Autodesk Inventor part; units mm, degrees
ref_plane "YZ Plane" through (0, 0, 0) normal (1, 0, 0) x (0, 1, 0)
ref_plane "XZ Plane" through (0, 0, 0) normal (0, 1, 0) x (-1, 0, 0)
ref_plane "XY Plane" through (0, 0, 0) normal (0, 0, 1) x (1, 0, 0)
sketch "Sketch1" plane through (0, 0, 0) normal (0, 1, 0) x (-1, 0, 0)
  line L0 (0, 0) -> (50, 0)
  line L1 (50, 0) -> (50, -60)
  line L2 (50, -60) -> (0, -60)
  line L3 (0, -60) -> (0, 0)
  dimension "d0" = 50
  dimension "d1" = 60
extrude "Extrusion1" add sketch "Sketch1" along normal blind 5
sketch "Sketch2" plane through (0, 5, 0) normal (0, 1, 0) x (1, 0, 0)
  line L0 (-50, 0) -> (0, 0)
  line L1 (-50, 60) -> (-50, 0)
  line L2 (0, 0) -> (-50, 0)
  line L3 (-50, 0) -> (-50, 40)
  line L4 (-50, 40) -> (0, 40)
  line L5 (0, 40) -> (0, 0)
  dimension "d4" = 40
extrude "Extrusion2" add sketch "Sketch2" along normal blind 11
sketch "Sketch3" plane through (0, 16, 0) normal (0, 1, 0) x (1, 0, 0)
  line L0 (0, 0) -> (-50, 0)
  line L1 (-50, 0) -> (-50, 60)
  line L2 (-50, 60) -> (0, 60)
  line L3 (0, 60) -> (0, 0)
extrude "Extrusion3" add sketch "Sketch3" along normal blind 5
sketch "Sketch4" plane through (0, 21, 0) normal (0, 1, 0) x (1, 0, 0)
  line L0 (0, 0) -> (0, 60)
  line L1 (-50, 40) -> (0, 40)
  line L2 (0, 60) -> (-50, 60)
  line L3 (-50, 60) -> (-50, 40)
  line L4 (-50, 40) -> (0, 40)
  line L5 (0, 40) -> (0, 60)
  line L6 (-50, 50) -> (0, 50)
  line L7 (-25, 50) -> (-50, 50)
  line L8 (-25, 50) -> (0, 50)
  circle A0 centre (-12.5, 50) radius 2.5
  circle A1 centre (-37.5, 50) radius 2.5
  dimension "d9" = 5
  dimension "d10" = 5
extrude "Extrusion4" cut sketch "Sketch4" against normal blind 5 contours A0 L6 | L6 A0 | A1 L6 | L6 A1
sketch "Sketch5" plane through (0, 21, 0) normal (0, 1, 0) x (1, 0, 0)
  line L0 (-50, 60) -> (-50, 0)
  line L1 (0, 0) -> (-50, 0)
  line L2 (-50, 0) -> (-50, 35)
  line L3 (-50, 35) -> (0, 35)
  line L4 (0, 35) -> (0, 0)
  line L5 (-37.5, 35) -> (-37.5, 0)
  line L6 (-12.5, 35) -> (-12.5, 0)
  dimension "d13" = 35
extrude "Extrusion5" add sketch "Sketch5" along normal blind 30 contours L3 L6 L1 L5
sketch "Sketch6" plane through (0, 51, 0) normal (0, 1, 0) x (1, 0, 0)
  line L0 (0, 0) -> (0, 60)
  line L1 (0, 0) -> (-49.8487, 0)
  line L2 (-49.8487, 0) -> (-49.8487, 35.2322)
  line L3 (-49.8487, 35.2322) -> (0, 35.2322)
  line L4 (0, 35.2322) -> (0, 0)
  line L5 (-49.8487, 17.6161) -> (0, 17.6161) construction
  line L6 (-24.9244, 0) -> (-24.9244, 35.2322) construction
  circle A0 centre (-24.9244, 17.6161) radius 5
  dimension "d16" = 10
extrude "Extrusion6" cut sketch "Sketch6" against normal blind 30 contours A0
sketch "Sketch7" plane through (0, 51, 0) normal (0, 1, 0) x (1, 0, 0)
  line L0 (-50, 35) -> (-50, 0)
  line L1 (0, 0) -> (-50, 0)
  line L2 (-50, 0) -> (-50, 35)
  line L3 (-50, 35) -> (0, 35)
  line L4 (0, 35) -> (0, 0)
  circle A0 centre (-24.9244, 17.6161) radius 5
  circle A1 centre (-24.9244, 17.6161) radius 5
  line L5 (-37.5, 35) -> (-37.5, 0)
  line L6 (-12.5, 35) -> (-12.5, 0)
extrude "Extrusion7" add sketch "Sketch7" along normal blind 10 contours L3 L6 L1 L5
chamfer "Chamfer1" distance 4 angle 45 1 edges at (-29.9244, 61, -17.6161)
sketch "Sketch8" plane through (0, 0, 0) normal (0, -1, 0) x (1, 0, 0)
  point P0 (0, 0)
sketch "Sketch9" plane through (0, 0, 0) normal (0, -1, 0) x (1, 0, 0)
  line L0 (0, -60) -> (-50, -60)
  line L1 (0, -60) -> (-15, -60)
  line L2 (-15, -60) -> (-15, -45)
  line L3 (-15, -45) -> (0, -45)
  line L4 (0, -45) -> (0, -60)
  line L5 (-50, -60) -> (-50, 0)
  line L6 (-50, -60) -> (-35, -60)
  line L7 (-35, -60) -> (-35, -45)
  line L8 (-35, -45) -> (-50, -45)
  line L9 (-50, -45) -> (-50, -60)
  line L10 (0, 0) -> (-15, 0)
  line L11 (-15, 0) -> (-15, -15)
  line L12 (-15, -15) -> (0, -15)
  line L13 (0, -15) -> (0, 0)
  line L14 (-50, 0) -> (-35, 0)
  line L15 (-35, 0) -> (-35, -15)
  line L16 (-35, -15) -> (-50, -15)
  line L17 (-50, -15) -> (-50, 0)
  point P0 (-50, -35)
  dimension "d24" = 15
  dimension "d25" = 15
  dimension "d26" = 15
  dimension "d27" = 15
  dimension "d28" = 15
  dimension "d29" = 15
extrude "Extrusion8" add sketch "Sketch9" along normal blind 12
fillet "Fillet1" radius 2 7 edges at (-25, 61, -35) (-25, 61, 0) (-25, 21, -60) (-25, 16, -60) (-25, 5, -60) (-12.5, 61, -17.5) (-37.5, 61, -17.5)
fillet "Fillet2" radius 1 10 edges at (-50, 20.4142, -59.4142) (-50, 18.5, -60) (-50, 16.5858, -59.4142) (-50, 16, -49) (-50, 21, -29) (0, 20.4142, -59.4142) (0, 18.5, -60) (0, 16.5858, -59.4142) (0, 16, -49) (0, 21, -29)
fillet "Fillet3" radius 1 16 edges at (-49.7071, 20.7071, 0) (-50, 4, 0) (-43.25, 21, 0) (-0.2929, 20.7071, 0) (0, 4, 0) (-6.75, 21, 0) (-50, 4.4142, -59.4142) (-50, 5, -49) (-50, -4.5, -60) (0, 4.4142, -59.4142) (0, 5, -49) (0, -4.5, -60) (0, 16.5, -40) (0, 10.5, -40) (-50, 16.5, -40) (-50, 10.5, -40)
fillet "Fillet4" radius 1 15 edges at (-13.0858, 60.4142, -0.5858) (-12.5, 40, 0) (-12.5, 20.5, 0) (-36.9142, 60.4142, -0.5858) (-37.5, 20.5, 0) (-37.5, 40, 0) (-13.0858, 60.4142, -34.4142) (-12.5, 40, -35) (-36.9142, 60.4142, -34.4142) (-37.5, 40, -35) (-37.5, 20.7071, -0.2929) (-37.5, 21, -18) (-25, 21, -35) (-12.5, 20.7071, -0.2929) (-12.5, 21, -18)
properties part number "PortaHerramienta1"
Read the model definition and answer for the solid it produces. Units are mm, in the model's axes. A direction names the side the tool comes from. Round coordinates to 2 decimals unless told otherwise and drop trailing zeros. Write each loop counter-clockwise with the first axis right and the second up, starting at its lowest first coordinate (ties: lowest second). Pieces come first, ordered by that corner, then holes. Notation, with made-up numbers: (25, -35.5) - (39, -35.5) arc R22 cw to (39, -15.5) - close; hole circle Ø1 at (89.25, 66). An arc over 180 degrees is marked (long way). One line per item, written item: value.
Q1. Find section A-A (z = -50). Determine the outline of the cut face in (x, y), and give its area (3 significant figures).
The answers:
outline: (-50, -12) - (-35, -12) - (-35, 0) - (-15, 0) - (-15, -12) - (0, -12) - (0, 4) arc R1 ccw to (-1, 5) - (-49, 5) arc R1 ccw to (-50, 4) - close; (-50, 17) arc R1 ccw to (-49, 16) - (-40, 16) - (-40, 21) - (-49, 21) arc R1 ccw to (-50, 20) - close; (-35, 16) - (-15, 16) - (-15, 21) - (-35, 21) - close; (-10, 16) - (-1, 16) arc R1 ccw to (0, 17) - (0, 20) arc R1 ccw to (-1, 21) - (-10, 21) - close
area: 809 mm2
Q2. Find section B-B (y = -7). Determine the outline of the cut face in (x, z), and give its area (3 significant figures).
The answers:
outline: (-50, -59) arc R1 ccw to (-49, -60) - (-35, -60) - (-35, -45) - (-50, -45) - close; (-50, -15) - (-35, -15) - (-35, 0) - (-49, 0) arc R1 ccw to (-50, -1) - close; (-15, -60) - (-1, -60) arc R1 ccw to (0, -59) - (0, -45) - (-15, -45) - close; (-15, -15) - (0, -15) - (0, -1) arc R1 ccw to (-1, 0) - (-15, 0) - close
area: 899 mm2
Q3. Which of the six approach directions +Z, -Z, +X, -X, +Y, -Y give full straight-line access (tool end or side, diameter ignored) to faces 5 (the cylindrical face through (-24.66, 4.4, -59.43)), 6 (the flat face through (-8, -6, -45)), 7 (the flat face through (-25, 40, -35)), 8 (the cylindrical face through (-35.19, 18.54, -49.04))?
The answers:
face 5: -Z, +X, -X
face 6: +X, -X, -Y
face 7: -Z, +X, -X, +Y
face 8: +Y
Q4. Each of these flat-tipped pins is pushed along its axis until it touches: P1, Ø8, axis at x = -24.92, z = -17.62, coming from the -Y side; P2, Ø5.5, axis at x = -34.5, z = -48.5, coming from the +Y side; P3, Ø9, axis at x = -16.5, y = 8.5, coming from the -Z side. Where does it stop, or does it pass through?
The answers:
P1: stops at y = 0
P2: stops at y = 21
P3: stops at z = -59.73
Q5. For a pull along Y with two mould halves and no side action, classify faces 1 (the cylindrical face through (-24.66, 16.57, -59.4)), 2 (the flat face through (-25, 16, -49)), 3 (the flat face through (-50, 4, -30)), 4 (the flat face through (-25.3, 21, -36.2)) as pulls with the +Y half, pulls with the -Y half, needs draft (parallel to the pull), parting line crosses it, or undercut.
The answers:
face 1: undercut
face 2: undercut
face 3: needs draft
face 4: pulls with the +Y half
Q6. Find section D-D (x = -43.5). Determine the outline of the cut face in (y, z), and give its area (3 significant figures).
The answers:
outline: (-12, -60) - (3, -60) arc R2 ccw to (5, -58) - (5, -40) - (16, -40) - (16, -58) arc R2 ccw to (18, -60) - (19, -60) arc R2 ccw to (21, -58) - (21, -1) arc R1 ccw to (20, 0) - (-12, 0) - (-12, -15) - (0, -15) - (0, -45) - (-12, -45) - close
area: 1,400 mm2
Q7. Straight lines are drawn through the part: line 1 (X direction, y = 19, z = -50); line 2 (Z direction, x = -5, y = -3.5); line 3 (Y direction, x = -40, z = -46.5). For each, find the intervals that lie inside material, in ascending order. Write a range as from..to.
The answers:
line 1: x = -50..-40, -35..-15, -10..0
line 2: z = -60..-45, -15..0
line 3: y = -12..5, 16..21
Q8. Find section C-C (z = -43). Determine the outline of the cut face in (x, y).
The answers:
outline: (-50, 0) - (0, 0) - (0, 4) arc R1 ccw to (-1, 5) - (-49, 5) arc R1 ccw to (-50, 4) - close; (-50, 17) arc R1 ccw to (-49, 16) - (-1, 16) arc R1 ccw to (0, 17) - (0, 20) arc R1 ccw to (-1, 21) - (-49, 21) arc R1 ccw to (-50, 20) - close
